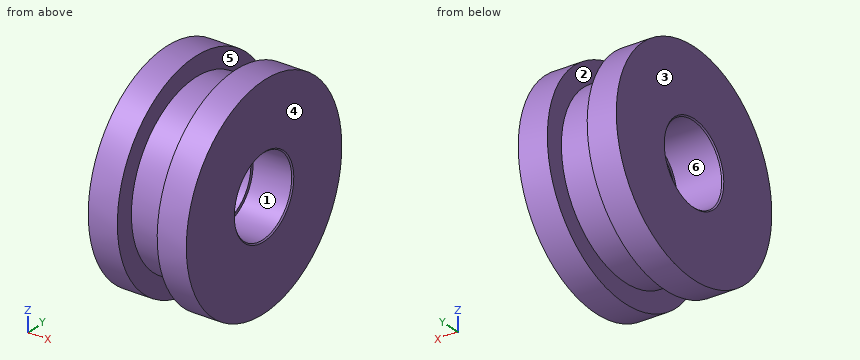
Solid Edge part; units mm, degrees
sketch "Sketch1" plane through (0, 0, 0) normal (0, -1, 0) x (1, 0, 0)
  line L0 (11.25, 17.5) -> (16, 17.5)
  line L1 (16, 17.5) -> (16, 6.5)
  line L2 (16, 6.5) -> (9.5, 6.5)
  line L3 (9.5, 6.5) -> (9.5, 6)
  line L4 (9.5, 6) -> (7.5, 6)
  line L5 (7.5, 6) -> (7.5, 6.5)
  line L6 (7.5, 6.5) -> (0, 6.5)
  line L7 (0, 6.5) -> (0, 17.5)
  line L8 (0, 17.5) -> (4.75, 17.5)
  line L9 (4.75, 17.5) -> (4.75, 14.34)
  line L10 (4.75, 14.34) -> (11.25, 14.34)
  line L11 (11.25, 14.34) -> (11.25, 17.5)
revolve "RevolvedProtrusion1" add sketch "Sketch1" angle 360 about axis through (0, 0, 0) along (1, 0, 0)
chamfer "Chamfer1" distance 0.2 angle 45 2 edges at (16, 0, -6.5) (0, 0, -6.5)
Geometry: final body of the model. Coordinates: model frame, mm. Face numbers are marked on the shaded views. A direction names the side the tool comes from. Coordinates: 2 decimals unless noted, no trailing zeros. Order: outer loops, then holes, each group sorted by start corner. A loop starts at its lowest first (then second) coordinate and runs counter-clockwise, first axis right, second up. Notation, with made-up numbers: (62.25, 13.25) - (77.25, 13.25) arc R26 cw to (77.25, 27.25) - close; hole circle Ø5 at (67, 50.25). An arc over 180 degrees is marked (long way). Return JSON: item names as keys, results as strings. Group by question number.
1. Set-up query: the marked faces 1, 2 and 3. Return all of +Z, -Z, +X, -X, +Y, -Y with unobstructed straight access to the full face (end or side cutting, diameter ignored); none if empty.
2. Material intervals for line 1 along Y through (x, z) = (4.5, 0); line 2 along X through (y, z) = (-4.5, 14); line 3 along Z through (x, y) = (8.3, 0), sorted ascending. Write a range as [from, to].
3. Cut plane C-C (x = 3.25). Output: boundary loops of the cut face in (y, z), plus the area to 3 significant figures.
4. Pull-direction query (X, two-part tool) for the marked faces 4, 5 and 6; classes: pulls with the +X half, pulls with the -X half, needs draft (parallel to the pull), parting line crosses it, or undercut.
5. Cut plane A-A (y = 0). Output: boundary loops of the cut face in (x, z).
6. Pin query (flat end, axial travel): pin 1 (6 mm diameter, centred on y = 1, z = 1.5, fed in from -X); pin 2 (2 mm diameter, centred on x = 10.5, z = -1.5, fed in from +Y); pin 3 (14.5 mm diameter, centred on y = -3, z = 1.5, fed in from +X); pin 4 (6 mm diameter, centred on x = 11.5, z = -6.5, fed in from +Y). Return the tip coordinate at first contact, or that it passes through.
7. Cut plane D-D (z = 13.5). Output: boundary loops of the cut face in (x, y), plus the area to 3 significant figures.
Resolved:
{
 "1": {"face 1": "+X", "face 2": "none", "face 3": "+Z, -Z, -X, +Y, -Y"},
 "2": {"line 1": "y = [-17.5, -6.5], [6.5, 17.5]", "line 2": "x = [0, 4.75], [11.25, 16]", "line 3": "z = [-14.34, -6], [6, 14.34]"},
 "3": {"outline": "circle Ø35 at (0, 0); hole circle Ø13 at (0, 0)", "area": "829 mm²"},
 "4": {"face 4": "pulls with the +X half", "face 5": "undercut", "face 6": "needs draft"},
 "5": {"outline": "(0, -17.5) - (4.75, -17.5) - (4.75, -14.34) - (11.25, -14.34) - (11.25, -17.5) - (16, -17.5) - (16, -6.7) - (15.8, -6.5) - (9.5, -6.5) - (9.5, -6) - (7.5, -6) - (7.5, -6.5) - (0.2, -6.5) - (0, -6.7) - close; (0, 6.7) - (0.2, 6.5) - (7.5, 6.5) - (7.5, 6) - (9.5, 6) - (9.5, 6.5) - (15.8, 6.5) - (16, 6.7) - (16, 17.5) - (11.25, 17.5) - (11.25, 14.34) - (4.75, 14.34) - (4.75, 17.5) - (0, 17.5) - close"},
 "6": {"pin 1": "passes through", "pin 2": "stops at y = 17.48", "pin 3": "stops at x = 16", "pin 4": "stops at y = 17.15"},
 "7": {"outline": "(0, -11.14) - (4.75, -11.14) - (4.75, -4.84) - (11.25, -4.84) - (11.25, -11.14) - (16, -11.14) - (16, 11.14) - (11.25, 11.14) - (11.25, 4.84) - (4.75, 4.84) - (4.75, 11.14) - (0, 11.14) - close", "area": "274 mm²"}
}
